Can you work these out from the model? Positions are in its coordinate system, mm. Face numbers are marked on the shaded views. A direction names the side the tool comes from. Round coordinates to 2 decimals unless told otherwise and drop trailing zeros. Order: outer loops, then holes, each group sorted by start corner. A loop starts at its lowest first (then second) coordinate and runs counter-clockwise, first axis right, second up. Notation, with made-up numbers: (-23.75, -14) -> (15.25, -14) arc R33 ccw to (15.25, 24) -> close; hole circle Ø10 at (42.25, 28.25). An arc over 180 degrees is marked (long way). One line per item, written item: value.
```python
from build123d import *

# Parameters (mm, degrees)
F0_R     = 31.75
F0_R_2   = 2.25
F1_DEPTH = 4
F2_R     = 31.75
F3_DEPTH = 8
F5_DEPTH = 8.89
F7_DEPTH = 20.891
F8_R     = 39.6924295133
F9_DEPTH = 4.318


with BuildPart() as f1:
    # F0 (on Front) → F1 (new body)
    with BuildSketch(Plane.XZ):
        Circle(F0_R)
        Circle(F0_R_2, mode=Mode.SUBTRACT)
    extrude(amount=F1_DEPTH)

    # F2 (on face) → F3 (join)
    with BuildSketch(Plane.XZ.offset(4)):
        Circle(F2_R)
        with BuildLine():
            ThreePointArc((2.25, 0), (-0.8345241318, -2.0895141716), (-1.630950643, 1.55))
            ThreePointArc((-1.630950643, 1.55), (0, 2.25), (1.630950643, 1.55))
            ThreePointArc((1.630950643, 1.55), (2.0895141716, 0.8345241318), (2.25, 0))
        make_face(mode=Mode.SUBTRACT)
        with BuildLine():
            ThreePointArc((1.630950643, 1.55), (0, 2.25), (-1.630950643, 1.55))
            Line((-1.630950643, 1.55), (1.630950643, 1.55))
        make_face()
    extrude(amount=F3_DEPTH)

    # F4 (on face) → F5 (join)
    with BuildSketch(Plane.XZ.offset(12)):
        with BuildLine():
            ThreePointArc((27.990753902, 14.986), (0, 31.75), (-27.990753902, 14.986))
            Line((-27.990753902, 14.986), (27.990753902, 14.986))
        make_face()
        with BuildLine():
            Line((27.990753902, -14.986), (-27.990753902, -14.986))
            ThreePointArc((-27.990753902, -14.986), (0, -31.75), (27.990753902, -14.986))
        make_face()
    extrude(amount=F5_DEPTH)

    # F6 (on face) → F7 (cut, through all)
    with BuildSketch(Plane.XZ.offset(20.89)):
        with BuildLine():
            Line((-27.990753902, -14.986), (-27.990753902, 14.986))
            ThreePointArc((-27.990753902, 14.986), (-31.75, 0), (-27.990753902, -14.986))
        make_face()
        with BuildLine():
            ThreePointArc((27.990753902, -14.986), (30.795851477, -7.7251557788), (31.75, 0))
            ThreePointArc((31.75, 0), (30.795851477, 7.7251557788), (27.990753902, 14.986))
            Line((27.990753902, 14.986), (27.990753902, -14.986))
        make_face()
    extrude(amount=-F7_DEPTH, mode=Mode.SUBTRACT)

    # F8 (on face) → F9 (cut)
    with BuildSketch(Plane(origin=(0, 0, 0), x_dir=(-1, 0, 0), z_dir=(0, 1, 0))):
        Circle(F8_R)
    extrude(amount=-F9_DEPTH, mode=Mode.SUBTRACT)


solid = f1.part
```
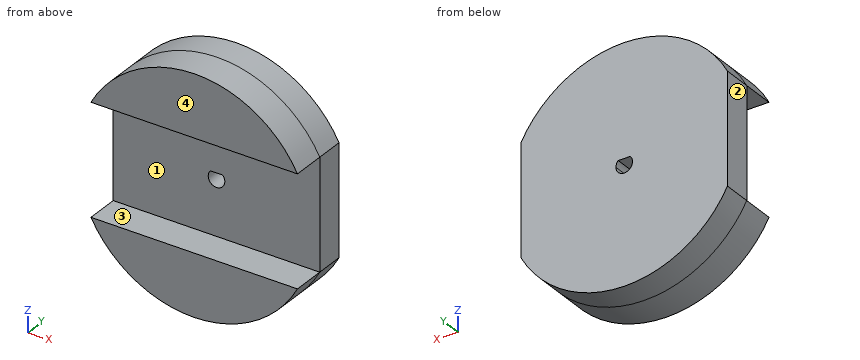
Q1. I want a section at A-A on y = -10. List the corners of the cut face in (x, z) for me, plus the area to 3 significant figures.
Answers below:
outline: (-27.99, -14.99) arc R31.75 ccw to (27.99, -14.99) -> (27.99, 14.99) arc R31.75 ccw to (-27.99, 14.99) -> close; hole (-1.63, 1.55) arc R2.25 ccw (long way) to (1.63, 1.55) -> close
area: 3,000 mm^2
Q2. Please list where these lines run through material, in increasing order: line 1 along Z through (x, y) = (0, -7.75); line 2 along Z through (x, y) = (-1, -12.75); line 3 along X through (y, z) = (-8.5, 0).
Answers below:
line 1: -31.75 to -2.25, 1.55 to 31.75
line 2: -31.73 to -14.99, 14.99 to 31.73
line 3: -27.99 to -2.25, 2.25 to 27.99
Q3. I want a section at D-D on z = -16. List the corners of the cut face in (x, y) for me, plus the area to 3 significant figures.
Answers below:
outline: (-27.42, -20.89) -> (27.42, -20.89) -> (27.42, -4.32) -> (-27.42, -4.32) -> close
area: 909 mm^2
Q4. We'd pull the mould along Z, two halves only. Please class the marked faces 1 and 2: released by +Z, released by -Z, zero draft, split by the parting line, or undercut.
Answers below:
face 1: undercut
face 2: zero draft
Q5. I want a section at C-C on y = -13.75. List the corners of the cut face in (x, z) for me.
Answers below:
outline: (-27.99, -14.99) arc R31.75 ccw to (27.99, -14.99) -> close; (-27.99, 14.99) -> (27.99, 14.99) arc R31.75 ccw to start
Q6. I want a section at B-B on x = 0. List the corners of the cut face in (y, z) for me, plus the area to 3 significant figures.
Answers below:
outline: (-20.89, -31.75) -> (-4.32, -31.75) -> (-4.32, -2.25) -> (-12, -2.25) -> (-12, -14.99) -> (-20.89, -14.99) -> close; (-20.89, 14.99) -> (-12, 14.99) -> (-12, 1.55) -> (-4.32, 1.55) -> (-4.32, 31.75) -> (-20.89, 31.75) -> close
area: 757 mm^2
Q7. Will these pins go through, and if not, where does the flat tip stop? pin 1 Ø9 at (x, z) = (2.5, -3) entering from -Y; pin 2 Ø4 at (y, z) = (-6.5, 20) entering from -X; pin 3 Ø3 at (y, z) = (-18.5, 15.5) entering from -X; pin 4 Ø2.5 at (x, z) = (0, 0) entering from -Y.
Answers below:
pin 1: y = -12
pin 2: x = -26.15
pin 3: x = -27.99
pin 4: through
Q8. On a 3-axis mill with a long thin cutter (end or side, diameter ignored), from which of +Z, -Z, +X, -X, +Y, -Y can I reach the whole of each face in a straight line? I mean the marked faces 3 and 4. Say none if no direction works.
Answers below:
face 3: +X, -X, -Y
face 4: +Z, -Z, +X, -X, -Y
